from build123d import *

# Parameters (mm, degrees)
F1_DEPTH = 63.5
F2_DEPTH = 25.4
F3_DEPTH = 7.9375
F5_R     = 6.35


with BuildPart() as f1:
    # F0 (on Front) → F1 (new body, symmetric)
    with BuildSketch(Plane.XZ):
        Polygon((41.275, -9.525), (41.275, 9.525), (22.225, 9.525), (-41.275, 9.525), (-41.275, -9.525), align=None)
    extrude(amount=F1_DEPTH, both=True)

    # F0 (on Front) → F2 (join, symmetric)
    with BuildSketch(Plane.XZ):
        with BuildLine():
            Line((22.225, 9.525), (41.275, 9.525))
            Line((41.275, 9.525), (41.275, 27.0002))
            ThreePointArc((41.275, 27.0002), (45.9246798487, 38.2255201513), (57.15, 42.8752))
            Line((57.15, 42.8752), (60.0982093367, 42.8752))
            Line((60.0982093367, 42.8752), (60.0982093367, 61.9252))
            Line((60.0982093367, 61.9252), (57.15, 61.9252))
            add(Edge.make_bspline(
                [(56.0381595364, 61.9074977439), (56.4108675509, 61.9161651955), (56.7815065443, 61.9220777941), (57.15, 61.9252)],
                knots=[110.4471262045, 110.4471262045, 110.4471262045, 110.4471262045, 111.5045361635, 111.5045361635, 111.5045361635, 111.5045361635], degree=3))
            ThreePointArc((56.0381595364, 61.9074977439), (32.064280425, 51.2996300016), (22.225, 27.0002))
            Line((22.225, 27.0002), (22.225, 9.525))
        make_face()
        Polygon((60.0982093367, 61.9252), (60.0982093367, 42.8752), (78.7747351631, 42.8752), (78.8008907845, 61.9252), align=None)
    extrude(amount=F2_DEPTH, both=True)

    # F0 (on Front) → F3 (join, symmetric)
    with BuildSketch(Plane.XZ):
        with BuildLine():
            Line((-41.275, 9.525), (22.225, 9.525))
            Line((22.225, 9.525), (22.225, 27.0002))
            ThreePointArc((22.225, 27.0002), (32.064280425, 51.2996300016), (56.0381595364, 61.9074977439))
            add(Edge.make_bspline(
                [(-41.275, 9.525), (-44.3938878809, 30.0415972741), (17.1085761993, 61.002177049), (56.0381595364, 61.9074977439)],
                knots=[0, 0, 0, 0, 110.4471262045, 110.4471262045, 110.4471262045, 110.4471262045], degree=3))
        make_face()
    extrude(amount=F3_DEPTH, both=True)

    # F0 (on Front) → F4 (revolve)
    with BuildSketch(Plane.XZ):
        Polygon((78.8008907845, 61.9252), (78.7747351631, 42.8752), (78.7681788206, 38.1), (110.8982093367, 38.1), (110.8982093367, 66.675), (78.8074122528, 66.675), align=None)
    revolve(axis=Axis((78.7877955367, 0, 52.3875), (0.0013729972, 0, 0.9999990574)))

    # F5
    f5_edges = [f1.edges().sort_by_distance(p)[0] for p in [
        (41.275, -63.5, 0),
        (-41.275, -63.5, 0),
        (41.275, 63.5, 0),
        (-41.275, 63.5, 0),
    ]]
    fillet(f5_edges, radius=F5_R)


solid = f1.part
Geometry: final body of the model. Coordinates: model frame, mm. A direction names the side the tool comes from. Round coordinates to 2 decimals unless told otherwise and drop trailing zeros. Loops run counter-clockwise (first coordinate to the right, second up) from the corner with the lowest first, then second, coordinate; pieces in that order, holes last. Notation, with made-up numbers: (-10, 26) - (44, 26) arc R11 ccw to (44, 32) - close; hole circle Ø3 at (-26, 23.25). An arc over 180 degrees is marked (long way). Write each question's results on one line, items separated by ' | '. Start each with the question number.
1) First-contact query: P1, Ø6, axis at x = -11.5, z = 15, coming from the -Y side; P2, Ø11, axis at x = 39, z = 25.5, coming from the +Y side; P3, Ø16.5, axis at x = -12.5, y = 37, coming from the +Z side (3 decimals). Flat tips, straight axial feed; report the tip coordinate or a pass-through.
2) Access query for faces 1 (the face through (22.225, 17, 18)), 2 (the face through (36, -25.4, 36)), 3 (the face through (39.464, -61.59, 0.133)). Directions: +Z, -Z, +X, -X, +Y, -Y. A direction counts if a zero-diameter tool reaches every point of the face in a straight line with its end or side. Return the directions, or none.
3) Mould query, pull axis X, two halves, no side actions, for faces 4 (the face through (41.275, -1, 4)), 5 (the face through (1, 35, 9.525)), 6 (the face through (-41.275, -1, 0)), 7 (the face through (44.047, -0.356, 35.962)). Classes: released by +X, released by -X, zero draft, split by the parting line, or undercut.
4) Cut plane B-B on y = -49.5. Return loops of the section in (x, z) (3 decimals), then the cut area to 3 significant figures.
5) Cut plane A-A on z = 7.5. Return loops of the section in (x, y) (3 decimals), then the cut area to 3 significant figures.
6) Line query: probe 1 along X at (y, z) = (-11, 15) (3 decimals); probe 2 along Z at (x, y) = (1.5, 31.5) (3 decimals); probe 3 along X at (y, z) = (-57, 6.5) (3 decimals). Output: solid intervals per line, ascending. Write a range as [from, to].
Verdict:
1) P1: stops at y = -7.94 | P2: stops at y = 25.4 | P3: stops at z = 9.525
2) face 1: +Z, -X, +Y | face 2: +Z, -X, -Y | face 3: +Z, -Z, +X, -Y
3) face 4: released by +X | face 5: zero draft | face 6: released by -X | face 7: undercut
4) outline: (-41.275, -9.525) - (41.275, -9.525) - (41.275, 9.525) - (-41.275, 9.525) - close | area: 1,570 mm2
5) outline: (-41.275, -57.15) arc R6.35 ccw to (-34.925, -63.5) - (34.925, -63.5) arc R6.35 ccw to (41.275, -57.15) - (41.275, 57.15) arc R6.35 ccw to (34.925, 63.5) - (-34.925, 63.5) arc R6.35 ccw to (-41.275, 57.15) - close | area: 10,400 mm2
6) probe 1: x = [22.225, 41.275] | probe 2: z = [-9.525, 9.525] | probe 3: x = [-41.275, 41.275]
